from build123d import *

# Parameters (mm, degrees)
BOSS_EXTRUDE1_DEPTH = 3.175
SKETCH3_R           = 2.5
CUT_EXTRUDE1_DEPTH  = 10


with BuildPart() as part:
    # Sketch2 → Boss-Extrude1 (new body)
    with BuildSketch(Plane(origin=(0, 0, 0), x_dir=(1, 0, 0), z_dir=(0, 1, 0))):
        with BuildLine():
            Line((21, 310), (21, 289))
            Line((21, 289), (21, 220))
            Line((21, 220), (40, 220))
            ThreePointArc((40, 220), (54.142135624, 214.142135624), (60, 200))
            Line((60, 200), (60, 110))
            ThreePointArc((60, 110), (54.142135624, 95.857864376), (40, 90))
            Line((40, 90), (21, 90))
            Line((21, 90), (21, 21))
            Line((21, 21), (21, 0))
            Line((21, 0), (319, 0))
            Line((319, 0), (319, 21))
            Line((319, 21), (319, 289))
            Line((319, 289), (319, 310))
            Line((319, 310), (21, 310))
        make_face()
    extrude(amount=BOSS_EXTRUDE1_DEPTH)

    # Sketch3 → Cut-Extrude1 (cut)
    with BuildSketch(Plane(origin=(0, 3.175, 0), x_dir=(1, 0, 0), z_dir=(0, 1, 0))):
        with Locations((41, 300)):
            Circle(SKETCH3_R)
        with Locations((10, 269)):
            Circle(SKETCH3_R)
        with Locations((299, 300)):
            Circle(SKETCH3_R)
        with Locations((330, 269)):
            Circle(SKETCH3_R)
        with Locations((330, 41)):
            Circle(SKETCH3_R)
        with Locations((299, 10)):
            Circle(SKETCH3_R)
        with Locations((41, 10)):
            Circle(SKETCH3_R)
        with Locations((10, 41)):
            Circle(SKETCH3_R)
    extrude(amount=-CUT_EXTRUDE1_DEPTH, mode=Mode.SUBTRACT)


solid = part.part
Input: part model. Units: mm. Frame: model coordinates. A direction names the side the tool comes from. Give positions to 0.01 mm unless a question says otherwise; leave off trailing zeros. Order: outer loops, then holes, each group sorted by start corner. A loop starts at its lowest first (then second) coordinate and runs counter-clockwise, first axis right, second up.
Q1. Draft query along Z for faces 1 (the cylindrical face through (54.297, 1.565, -96.014)), 2 (the flat face through (168, 0, -157)). Return one class per face: +Z half, -Z half, draft (parallel to the pull), parting line (faces both ways), or undercut.
Checked values:
face 1: undercut
face 2: draft
Q2. Section A-A on y = 1.6. Output: boundary loops of the cut face in (x, z).
Checked values:
outline: (21, -310) - (319, -310) - (319, 0) - (21, 0) - (21, -90) - (40, -90) arc R20 cw to (60, -110) - (60, -200) arc R20 cw to (40, -220) - (21, -220) - close; hole circle Ø5 at (41, -300); hole circle Ø5 at (41, -10); hole circle Ø5 at (299, -300); hole circle Ø5 at (299, -10)
Q3. Set-up query: faces 3 (the cylindrical face through (53.986, 1.565, -214.297)), 4 (the flat face through (168, 3.175, -157)). Return all of +Z, -Z, +X, -X, +Y, -Y with unobstructed straight access to the full face (end or side cutting, diameter ignored); none if empty.
Checked values:
face 3: -X, +Y, -Y
face 4: +Z, -Z, +X, -X, +Y
Q4. Section B-B on z = -187. Output: boundary loops of the cut face in (x, y) (3 decimals), and give its area (3 significant figures).
Checked values:
outline: (60, 0) - (319, 0) - (319, 3.175) - (60, 3.175) - close
area: 822 mm2
Q5. Ray query, probe 1 along X at (y, z) = (0.95, -10); probe 2 along Z at (x, y) = (299, 2.05); probe 3 along Z at (x, y) = (41, 1.35). Return the intervals inside material, ascending.
Checked values:
probe 1: x = 21 to 38.5, 43.5 to 296.5, 301.5 to 319
probe 2: z = -310 to -302.5, -297.5 to -12.5, -7.5 to 0
probe 3: z = -310 to -302.5, -297.5 to -219.97, -90.03 to -12.5, -7.5 to 0
Q6. Contact query for flat-ended pins moving along their axis: pin 1 Ø4.5 at (x, z) = (299, -10) entering from +Y; pin 2 Ø1 at (y, z) = (1.5, -170.5) entering from -X. Output: stop coordinate, or through.
Checked values:
pin 1: passes through
pin 2: stops at x = 60
